Geometry: final body of the model. Coordinates: model frame, mm. Face numbers are marked on the shaded views. A direction names the side the tool comes from. Give positions to 0.01 mm unless a question says otherwise; leave off trailing zeros. Write each loop counter-clockwise with the first axis right and the second up, starting at its lowest first coordinate (ties: lowest second). Pieces come first, ordered by that corner, then holes. Notation, with made-up numbers: (-37, 33.25) -> (-28, 33.25) arc R36 cw to (-28, 72.25) -> close; hole circle Ø6 at (55.5, 30.5). An arc over 180 degrees is marked (long way). Answer as a JSON object with one key per item and string values.
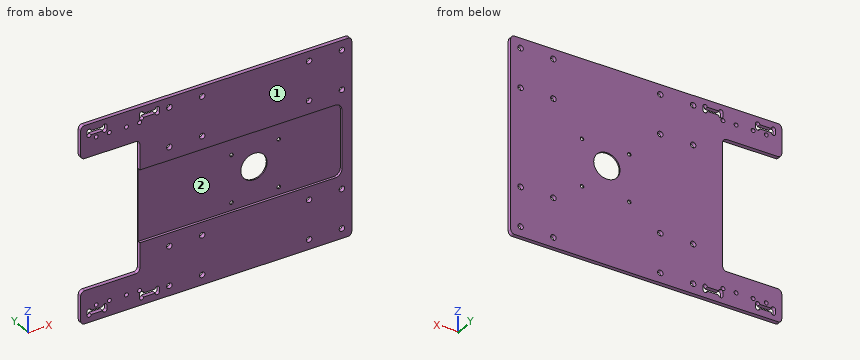
from build123d import *

# Parameters (mm, degrees)
SKETCH_1_W          = 206.4
SKETCH_1_H          = 150
SKETCH_1_R          = 2.1
SKETCH_1_R_2        = 1.5
EXTRUDE_1_DEPTH     = 3
CUT_EXTRUDE_1_DEPTH = 153.892903694
FILLET_1_R          = 3
CUT_EXTRUDE_2_DEPTH = 2
SKETCH_6_R          = 10
CUT_EXTRUDE_3_DEPTH = 10
SKETCH_7_W          = 45
SKETCH_7_H          = 100
CUT_EXTRUDE_4_DEPTH = 10
FILLET_2_R          = 3
CUT_EXTRUDE_5_DEPTH = 10


with BuildPart() as part:
    # 草图1 → 凸台-拉伸1 (new body)
    with BuildSketch(Plane(origin=(0, 0, 0), x_dir=(1, 0, 0), z_dir=(0, 1, 0))):
        with Locations((-30, 0)):
            Rectangle(SKETCH_1_W, SKETCH_1_H)
        with Locations(Location((65.7, 67.5, 0), (0, 0, 270))):
            Circle(SKETCH_1_R, mode=Mode.SUBTRACT)
        with Locations(Location((65.7, -67.5, 0), (0, 0, 90))):
            Circle(SKETCH_1_R, mode=Mode.SUBTRACT)
        with Locations(Location((-65.7, -67.5, 0), (0, 0, 270))):
            Circle(SKETCH_1_R, mode=Mode.SUBTRACT)
        with Locations(Location((-65.7, 67.5, 0), (0, 0, 90))):
            Circle(SKETCH_1_R, mode=Mode.SUBTRACT)
        with Locations(Location((-65.7, 37.5, 0), (0, 0, 270))):
            Circle(SKETCH_1_R, mode=Mode.SUBTRACT)
        with Locations(Location((-40.7, 37.5, 0), (0, 0, 270))):
            Circle(SKETCH_1_R, mode=Mode.SUBTRACT)
        with Locations(Location((-40.7, 67.5, 0), (0, 0, 270))):
            Circle(SKETCH_1_R, mode=Mode.SUBTRACT)
        with Locations(Location((-40.7, -67.5, 0), (0, 0, 270))):
            Circle(SKETCH_1_R, mode=Mode.SUBTRACT)
        with Locations(Location((-40.7, -37.5, 0), (0, 0, 270))):
            Circle(SKETCH_1_R, mode=Mode.SUBTRACT)
        with Locations(Location((-65.7, -37.5, 0), (0, 0, 270))):
            Circle(SKETCH_1_R, mode=Mode.SUBTRACT)
        with Locations(Location((40.7, -67.5, 0), (0, 0, 270))):
            Circle(SKETCH_1_R, mode=Mode.SUBTRACT)
        with Locations(Location((40.7, -37.5, 0), (0, 0, 270))):
            Circle(SKETCH_1_R, mode=Mode.SUBTRACT)
        with Locations(Location((65.7, -37.5, 0), (0, 0, 270))):
            Circle(SKETCH_1_R, mode=Mode.SUBTRACT)
        with Locations(Location((65.7, 37.5, 0), (0, 0, 270))):
            Circle(SKETCH_1_R, mode=Mode.SUBTRACT)
        with Locations(Location((40.7, 37.5, 0), (0, 0, 270))):
            Circle(SKETCH_1_R, mode=Mode.SUBTRACT)
        with Locations(Location((40.7, 67.5, 0), (0, 0, 270))):
            Circle(SKETCH_1_R, mode=Mode.SUBTRACT)
        with Locations(Location((-98.4, 63.575, 0), (0, 0, 270))):
            Circle(SKETCH_1_R_2, mode=Mode.SUBTRACT)
        with Locations(Location((-88.4, 63.575, 0), (0, 0, 270))):
            Circle(SKETCH_1_R_2, mode=Mode.SUBTRACT)
        with Locations(Location((-111.4, 63.575, 0), (0, 0, 270))):
            Circle(SKETCH_1_R_2, mode=Mode.SUBTRACT)
        with Locations(Location((-121.4, 63.575, 0), (0, 0, 270))):
            Circle(SKETCH_1_R_2, mode=Mode.SUBTRACT)
        with Locations(Location((-121.4, -63.474999999, 0), (0, 0, 270))):
            Circle(SKETCH_1_R_2, mode=Mode.SUBTRACT)
        with Locations(Location((-111.4, -63.474999999, 0), (0, 0, 270))):
            Circle(SKETCH_1_R_2, mode=Mode.SUBTRACT)
        with Locations(Location((-98.4, -63.425, 0), (0, 0, 270))):
            Circle(SKETCH_1_R_2, mode=Mode.SUBTRACT)
        with Locations(Location((-88.4, -63.425, 0), (0, 0, 270))):
            Circle(SKETCH_1_R_2, mode=Mode.SUBTRACT)
    extrude(amount=EXTRUDE_1_DEPTH)

    # 草图2 → 切除-拉伸1 (cut, through all)
    with BuildSketch(Plane(origin=(0, 0, 0), x_dir=(1, 0, 0), z_dir=(0, 1, 0))):
        with BuildLine():
            Line((-125.2, -66.425), (-116.5, -66.425))
            ThreePointArc((-116.5, -66.425), (-114.9, -64.825), (-113.3, -66.425))
            Line((-113.3, -66.425), (-113.3, -69.575))
            ThreePointArc((-113.3, -69.575), (-114.9, -71.175), (-116.5, -69.575))
            Line((-116.5, -69.575), (-125.2, -69.575))
            ThreePointArc((-125.2, -69.575), (-126.8, -71.175), (-128.4, -69.575))
            Line((-128.4, -69.575), (-128.4, -66.425))
            ThreePointArc((-128.4, -66.425), (-126.8, -64.825), (-125.2, -66.425))
        make_face()
        with BuildLine():
            Line((-85.2, -66.425), (-76.5, -66.425))
            ThreePointArc((-76.5, -66.425), (-74.9, -64.825), (-73.3, -66.425))
            Line((-73.3, -66.425), (-73.3, -69.575))
            ThreePointArc((-73.3, -69.575), (-74.9, -71.175), (-76.5, -69.575))
            Line((-76.5, -69.575), (-85.2, -69.575))
            ThreePointArc((-85.2, -69.575), (-86.8, -71.175), (-88.4, -69.575))
            Line((-88.4, -69.575), (-88.4, -66.425))
            ThreePointArc((-88.4, -66.425), (-86.8, -64.825), (-85.2, -66.425))
        make_face()
        with BuildLine():
            Line((-73.3, 66.425), (-73.3, 69.575))
            ThreePointArc((-73.3, 69.575), (-74.9, 71.175), (-76.5, 69.575))
            Line((-76.5, 69.575), (-85.2, 69.575))
            ThreePointArc((-85.2, 69.575), (-86.8, 71.175), (-88.4, 69.575))
            Line((-88.4, 69.575), (-88.4, 66.425))
            ThreePointArc((-88.4, 66.425), (-86.8, 64.825), (-85.2, 66.425))
            Line((-85.2, 66.425), (-76.5, 66.425))
            ThreePointArc((-76.5, 66.425), (-74.9, 64.825), (-73.3, 66.425))
        make_face()
        with BuildLine():
            Line((-113.3, 66.425), (-113.3, 69.575))
            ThreePointArc((-113.3, 69.575), (-114.9, 71.175), (-116.5, 69.575))
            Line((-116.5, 69.575), (-125.2, 69.575))
            ThreePointArc((-125.2, 69.575), (-126.8, 71.175), (-128.4, 69.575))
            Line((-128.4, 69.575), (-128.4, 66.425))
            ThreePointArc((-128.4, 66.425), (-126.8, 64.825), (-125.2, 66.425))
            Line((-125.2, 66.425), (-116.5, 66.425))
            ThreePointArc((-116.5, 66.425), (-114.9, 64.825), (-113.3, 66.425))
        make_face()
    extrude(amount=CUT_EXTRUDE_1_DEPTH, mode=Mode.SUBTRACT)

    # 圆角1
    fillet_1_edges = [part.edges().sort_by_distance(p)[0] for p in [
        (73.2, 1.5, 75),
        (-133.2, 1.5, 75),
        (-133.2, 1.5, -75),
        (73.2, 1.5, -75),
    ]]
    fillet(fillet_1_edges, radius=FILLET_1_R)

    # 草图4 → 切除-拉伸2 (cut)
    with BuildSketch(Plane(origin=(0, 0, 0), x_dir=(1, 0, 0), z_dir=(0, 1, 0))):
        with BuildLine():
            Line((-120.7, -27.5), (60.7, -27.5))
            ThreePointArc((60.7, -27.5), (64.235533906, -26.035533906), (65.7, -22.5))
            Line((65.7, -22.5), (65.7, 22.5))
            ThreePointArc((65.7, 22.5), (64.235533906, 26.035533906), (60.7, 27.5))
            Line((60.7, 27.5), (-120.7, 27.5))
            ThreePointArc((-120.7, 27.5), (-124.235533906, 26.035533906), (-125.7, 22.5))
            Line((-125.7, 22.5), (-125.7, -22.5))
            ThreePointArc((-125.7, -22.5), (-124.235533906, -26.035533906), (-120.7, -27.5))
        make_face()
    extrude(amount=CUT_EXTRUDE_2_DEPTH, mode=Mode.SUBTRACT)

    # 草图6 → 切除-拉伸3 (cut)
    with BuildSketch(Plane(origin=(0, 3, 0), x_dir=(1, 0, 0), z_dir=(0, 1, 0))):
        with Locations(Location((0, 0, 0), (0, 0, 270))):
            Circle(SKETCH_6_R)
    extrude(amount=-CUT_EXTRUDE_3_DEPTH, mode=Mode.SUBTRACT)

    # 草图7 → 切除-拉伸4 (cut)
    with BuildSketch(Plane(origin=(0, 3, 0), x_dir=(1, 0, 0), z_dir=(0, 1, 0))):
        with Locations((-110.7, 0)):
            Rectangle(SKETCH_7_W, SKETCH_7_H)
    extrude(amount=-CUT_EXTRUDE_4_DEPTH, mode=Mode.SUBTRACT)

    # 圆角2
    fillet_2_edges = [part.edges().sort_by_distance(p)[0] for p in [
        (-133.2, 1.5, 50),
        (-133.2, 1.5, -50),
        (-88.2, 1.5, -50),
        (-88.2, 1.5, 50),
    ]]
    fillet(fillet_2_edges, radius=FILLET_2_R)

    # 草图8 → 切除-拉伸5 (cut)
    with BuildSketch(Plane.XZ.offset(-2)):
        with BuildLine():
            ThreePointArc((17.542961637, 14.384893438), (18.892961637, 13.034893438), (20.242961637, 14.384893438))
            ThreePointArc((20.242961637, 14.384893438), (18.892961637, 15.734893438), (17.542961637, 14.384893438))
        make_face()
        with BuildLine():
            ThreePointArc((-18.457038363, 14.384893438), (-17.107038363, 13.034893438), (-15.757038363, 14.384893438))
            ThreePointArc((-15.757038363, 14.384893438), (-17.107038363, 15.734893438), (-18.457038363, 14.384893438))
        make_face()
        with BuildLine():
            ThreePointArc((-15.757038363, -21.615106562), (-17.107038363, -20.265106562), (-18.457038363, -21.615106562))
            ThreePointArc((-18.457038363, -21.615106562), (-17.107038363, -22.965106562), (-15.757038363, -21.615106562))
        make_face()
        with BuildLine():
            ThreePointArc((20.242961637, -21.615106562), (18.892961637, -20.265106562), (17.542961637, -21.615106562))
            ThreePointArc((17.542961637, -21.615106562), (18.892961637, -22.965106562), (20.242961637, -21.615106562))
        make_face()
    extrude(amount=-CUT_EXTRUDE_5_DEPTH, mode=Mode.SUBTRACT)


solid = part.part
Q1. Set-up query: the marked faces 1 and 2. Return all of +Z, -Z, +X, -X, +Y, -Y with unobstructed straight access to the full face (end or side cutting, diameter ignored); none if empty.
Values:
{"face 1": "+Z, -Z, +X, -X, -Y", "face 2": "-X, -Y"}
Q2. Material intervals for L1, parallel to Z at x = -121.4, y = 0.9 (3 decimals); L2, parallel to Z at x = -119, y = 1.65 (3 decimals); L3, parallel to Z at x = 31, y = 0.55, sorted ascending. Write a range as from..to.
Values:
{"L1": "-75..-69.575, -66.425..-65.075, -62.075..-50, 50..61.975, 64.975..66.425, 69.575..75", "L2": "-75..-69.575, -66.425..-50, 50..66.425, 69.575..75", "L3": "-75..-27.5, 27.5..75"}
Q3. Cut plane B-B (x = -102). Return the cut outline in (y, z), and give its area (3 significant figures).
Values:
{"outline": "(0, -75) -> (3, -75) -> (3, -50) -> (0, -50) -> close; (0, 50) -> (3, 50) -> (3, 75) -> (0, 75) -> close", "area": "150 mm²"}
Q4. First-contact query: P1, Ø3.5, axis at x = -98.4, z = -63.575, coming from the -Y side. Flat tip, straight axial feed; report the tip coordinate or a pass-through.
Values:
{"P1": "y = 0"}
Q5. Cut plane D-D (y = 1.5). State how many separate pieces and enclosed holes the cut face has, and give its area (3 significant figures).
Values:
{"separate pieces": "1", "enclosed holes": "28", "area": "17,500 mm²"}
Q6. Cut plane A-A (x = -40.7). Return the cut outline in (y, z).
Values:
{"outline": "(0, -75) -> (3, -75) -> (3, -69.6) -> (0, -69.6) -> close; (0, -65.4) -> (3, -65.4) -> (3, -39.6) -> (0, -39.6) -> close; (0, -35.4) -> (3, -35.4) -> (3, 35.4) -> (0, 35.4) -> (0, 27.5) -> (2, 27.5) -> (2, -27.5) -> (0, -27.5) -> close; (0, 39.6) -> (3, 39.6) -> (3, 65.4) -> (0, 65.4) -> close; (0, 69.6) -> (3, 69.6) -> (3, 75) -> (0, 75) -> close"}
Q7. Cut plane C-C (z = 0). Return the cut outline in (x, y), and give its area (3 significant figures).
Values:
{"outline": "(-88.2, 2) -> (-10, 2) -> (-10, 3) -> (-88.2, 3) -> close; (10, 2) -> (65.7, 2) -> (65.7, 0) -> (73.2, 0) -> (73.2, 3) -> (10, 3) -> close", "area": "156 mm²"}
